Can you work these out from the model? Positions are in its coordinate system, mm. A direction names the side the tool comes from. Give positions to 0.01 mm unless a question says otherwise; leave off trailing zeros. Loops run counter-clockwise (first coordinate to the right, second up) from the corner with the lowest first, then second, coordinate; pieces in that order, holes last.
from build123d import *

# Parameters (mm, degrees)
ESQUISSE1_R             = 25
BOSS_EXTRU_1_DEPTH      = 3
ESQUISSE3_R             = 6
BOSS_EXTRU_3_DEPTH      = 9
ESQUISSE4_R             = 5
ENL_V_MAT_EXTRU_2_DEPTH = 5


with BuildPart() as part:
    # Esquisse1 → Boss.-Extru.1 (new body)
    with BuildSketch(Plane.XY):
        Circle(ESQUISSE1_R)
    extrude(amount=BOSS_EXTRU_1_DEPTH)

    # Esquisse3 → Boss.-Extru.3 (add)
    with BuildSketch(Plane(origin=(0, 0, 0), x_dir=(-1, 0, 0), z_dir=(0, 0, -1))):
        Circle(ESQUISSE3_R)
        with BuildLine():
            Line((-1.397318861, 1.5), (1.397318861, 1.5))
            ThreePointArc((1.397318861, 1.5), (0, -2.05), (-1.397318861, 1.5))
        make_face(mode=Mode.SUBTRACT)
    extrude(amount=BOSS_EXTRU_3_DEPTH)

    # Esquisse4 → Enlèv. mat.-Extru.2 (cut)
    with BuildSketch(Plane.XY.offset(3)):
        with Locations((-8.295445994, -14.94087289)):
            Circle(ESQUISSE4_R)
    extrude(amount=-ENL_V_MAT_EXTRU_2_DEPTH, mode=Mode.SUBTRACT)


solid = part.part
(1) Please list where these lines run through material, in increasing order: probe 1 along Z at (x, y) = (8, 9); probe 2 along Y at (x, z) = (0.5, -6); probe 3 along Y at (x, z) = (-11.5, 1.25).
Returned:
probe 1: z = 0 to 3
probe 2: y = -5.98 to -1.99, 1.5 to 5.98
probe 3: y = -22.2 to -18.78, -11.1 to 22.2
(2) Thinking about a two-plate mould opening in X: for faces 3 (the flat face through (-3, 0, -9)), 4 (the cylindrical face through (6, 0, -4)), 5 (the cylindrical face through (-0.07, -2.05, -4.44)), which applies, pulls with the +X half, pulls with the -X half, needs draft (parallel to the pull), parting line crosses it, or undercut?
Returned:
face 3: needs draft
face 4: parting line crosses it
face 5: undercut
(3) Suppose I cut it at C-C on z = -6.25. List the corners of the cut face in (x, y) for me.
Returned:
outline: circle Ø12 at (0, 0); hole (-1.4, 1.5) arc R2.05 ccw (long way) to (1.4, 1.5) - close
(4) Will these pins go through, and if not, where does the flat tip stop? P1, Ø3, axis at x = -0.5, z = -6, coming from the -Y side; P2, Ø8, axis at x = 6.5, y = -15, coming from the -Z side; P3, Ø3, axis at y = -10, z = 1, coming from the +X side.
Returned:
P1: stops at y = -6
P2: stops at z = 0
P3: stops at x = 23.51
(5) Which directions (+Z, -Z, +X, -X, +Y, -Y) give clear straight access to the entire face, cutting with the end or side of a thin tool? Please do faces 1 (the cylindrical face through (23.846, 7.509, 1.479)), 2 (the flat face through (5, 6, 0)).
Returned:
face 1: +Z, -Z
face 2: -Z
(6) Suppose I cut it at A-A on y = 0. List the corners of the cut face in (x, z) for me.
Returned:
outline: (-25, 0) - (-6, 0) - (-6, -9) - (-2.05, -9) - (-2.05, 0) - (2.05, 0) - (2.05, -9) - (6, -9) - (6, 0) - (25, 0) - (25, 3) - (-25, 3) - close
(7) Suppose I cut it at B-B on x = 0. List the corners of the cut face in (y, z) for me, plus the area to 3 significant figures.
Returned:
outline: (-25, 0) - (-6, 0) - (-6, -9) - (-2.05, -9) - (-2.05, 0) - (1.5, 0) - (1.5, -9) - (6, -9) - (6, 0) - (25, 0) - (25, 3) - (-25, 3) - close
area: 226 mm2
(8) Suppose I cut it at D-D on y = 11. List the corners of the cut face in (x, z) for me.
Returned:
outline: (-22.45, 0) - (22.45, 0) - (22.45, 3) - (-22.45, 3) - close
